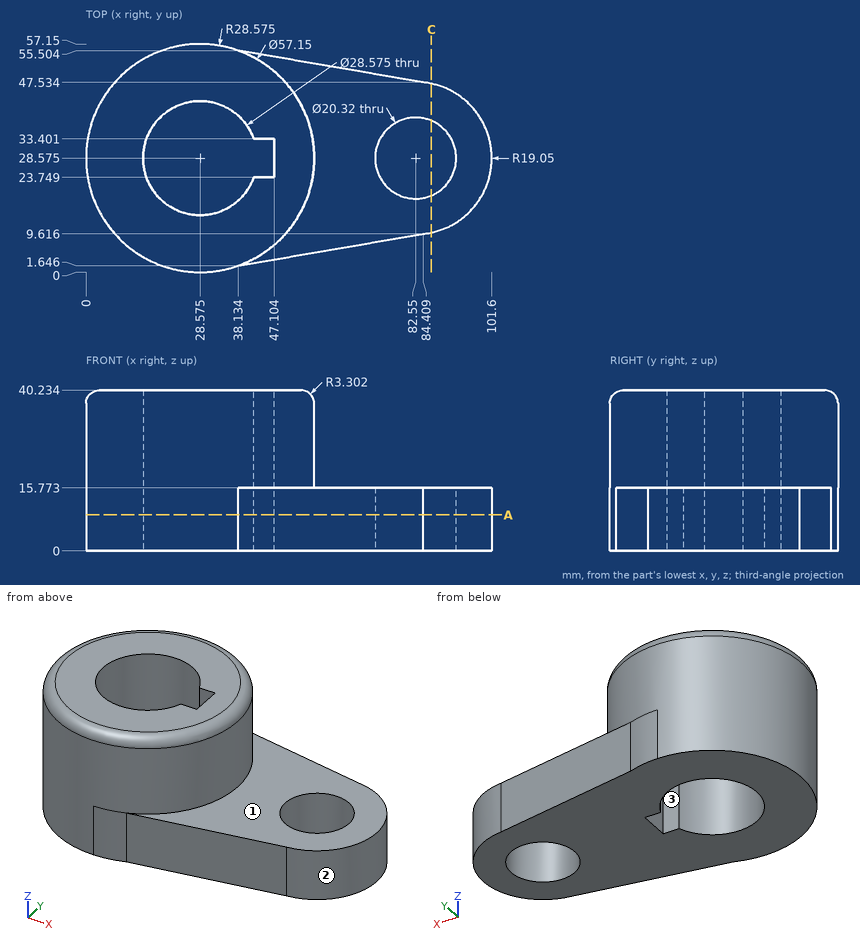
Can you work these out from the drawing? Everything is in mm from the part's minimum corner. Give positions to 0.01 mm unless a question says otherwise; leave off trailing zeros. Order: outer loops, then holes, each group sorted by start corner. A loop starts at its lowest first (then second) coordinate and runs counter-clockwise, first axis right, second up. Notation, with made-up numbers: M 24.25,-10 L 34.25,-10 A15 ccw 34.25,-1 Z; hole C 61.25,32.25 d7. An arc over 180 degrees is marked long. Write item = value, one per line. Start each with the question number.
Q1. Suppose I cut it at A-A (z = 9). Count the separate pieces of the cut face and the enclosed holes in it, plus the area to 3 significant figures.
Q2. I need wall thicknesses on probe 1 along X at (y, z) = (25, 9) (1 decimal); probe 2 along X at (y, z) = (33, 26) (1 decimal); probe 3 along X at (y, z) = (33, 10.5) (1 decimal). Which ranges of each line are inside material? Lowest first, please. Write a range as [from, to].
Q3. Will these pins go through, and if not, where does the flat tip stop? pin 1 Ø2 at (x, z) = (22.5, 32) entering from -Y; pin 2 Ø3 at (y, z) = (8.5, 33.5) entering from +X; pin 3 Ø1 at (x, z) = (69, 6) entering from -Y; pin 4 Ø23.5 at (x, y) = (82.55, 28.575) entering from -Z.
Q4. We'd pull the mould along X, two halves only. Please class the marked faces 1, 2 and 3: pulls with the +X half, pulls with the -X half, needs draft (parallel to the pull), parting line crosses it, or undercut.
Q5. Suppose I cut it at C-C (x = 86.5). Write out the boundary of the cut face in (y, z) (1 decimal).
Check result:
q1.separate_pieces = 1
q1.enclosed_holes = 2
q1.area = 3,430 mm2
q2.probe_1 = [0.2, 14.7], [47.1, 73], [92.1, 101.3]
q2.probe_2 = [0.3, 15], [47.1, 56.8]
q2.probe_3 = [0.3, 15], [47.1, 73.4], [91.7, 101.1]
q3.pin_1 = 0.45
q3.pin_2 = 50.29
q3.pin_3 = 6.88
q3.pin_4 = 0
q4.face_1 = needs draft
q4.face_2 = pulls with the +X half
q4.face_3 = undercut
q5.outline = M 9.9,0 L 19.2,0 L 19.2,15.8 L 9.9,15.8 Z; M 37.9,0 L 47.2,0 L 47.2,15.8 L 37.9,15.8 Z
